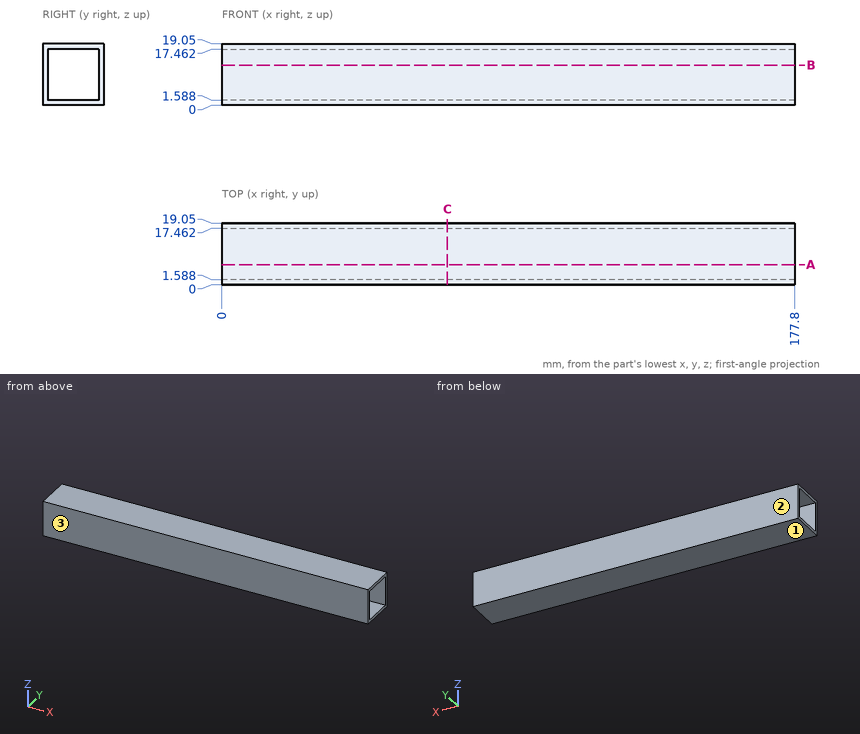
Check sheet for the drawn part. Datum: minimum x, y, z corner. Units: mm. Round coordinates to 2 decimals unless told otherwise and drop trailing zeros. Order: outer loops, then holes, each group sorted by start corner. A loop starts at its lowest first (then second) coordinate and runs counter-clockwise, first axis right, second up.
1) Section check A-A (y = 6.25). Record the boundary of the cut face in (x, z).
2) Scan line: line 1 (Y direction, x = 43, z = 12.5). Record every from-to range of solid material in increasing order.
3) Mould release check, pull along Y, two halves, no side actions. Record for the marked faces 1, 2 and 3: +Y half, -Y half, draft (parallel to the pull), parting line (faces both ways), or undercut.
4) Section check C-C (x = 70). Record the boundary of the cut face in (y, z), and give its area (3 significant figures).
Result:
1. outline: (0, 0) - (177.8, 0) - (177.8, 1.59) - (0, 1.59) - close; (0, 17.46) - (177.8, 17.46) - (177.8, 19.05) - (0, 19.05) - close
2. line 1: y = 0 to 1.59, 17.46 to 19.05
3. face 1: draft
3. face 2: +Y half
3. face 3: -Y half
4. outline: (0, 0) - (19.05, 0) - (19.05, 19.05) - (0, 19.05) - close; hole (1.59, 1.59) - (17.46, 1.59) - (17.46, 17.46) - (1.59, 17.46) - close
4. area: 111 mm2
